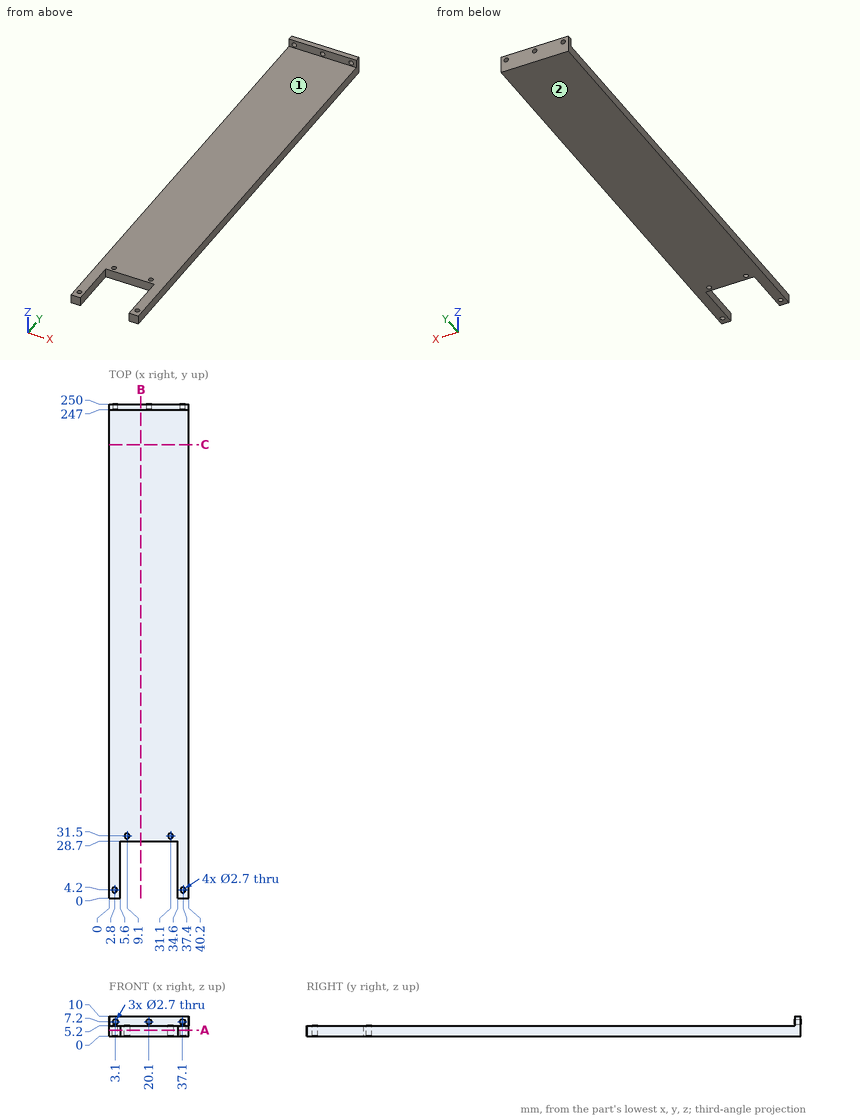
Source: three-view drawing plus pictorial views. Frame: mm from the lowest corner of the part. A direction names the side the tool comes from. Coordinates: 2 decimals unless noted, no trailing zeros. Order: outer loops, then holes, each group sorted by start corner. A loop starts at its lowest first (then second) coordinate and runs counter-clockwise, first axis right, second up.
1) Section B-B (x = 16). Return loops of the section in (y, z), then the cut area to 3 significant figures.
Result sheet:
outline: (28.7, 0) - (250, 0) - (250, 10) - (247, 10) - (247, 5.2) - (28.7, 5.2) - close
area: 1,170 mm2
2) Section A-A (z = 3). Return loops of the section in (x, y).
Result sheet:
outline: (0, 0) - (5.6, 0) - (5.6, 28.7) - (34.6, 28.7) - (34.6, 0) - (40.2, 0) - (40.2, 250) - (0, 250) - close; hole circle Ø2.7 at (2.8, 4.2); hole circle Ø2.7 at (9.1, 31.5); hole circle Ø2.7 at (31.1, 31.5); hole circle Ø2.7 at (37.4, 4.2)
3) Section C-C (y = 229.5). Return loops of the section in (x, z), then the cut area to 3 significant figures.
Result sheet:
outline: (0, 0) - (40.2, 0) - (40.2, 5.2) - (0, 5.2) - close
area: 209 mm2
4) Ray query, probe 1 along Z at (x, y) = (37.1, 248.3); probe 2 along Y at (x, z) = (37.4, 1.1); probe 3 along Y at (x, z) = (9.1, 2.4). Return the intervals inside material, ascending.
Result sheet:
probe 1: z = 0 to 5.85, 8.55 to 10
probe 2: y = 0 to 2.85, 5.55 to 250
probe 3: y = 28.7 to 30.15, 32.85 to 250
5) First-contact query: P1, Ø1.6, axis at x = 19, z = 3.5, coming from the -Y side; P2, Ø6, axis at x = 16, y = 135, coming from the +Z side; P3, Ø5.5, axis at x = 25, z = 8, coming from the -Y side. Flat tips, straight axial feed; report the tip coordinate or a pass-through.
Result sheet:
P1: stops at y = 28.7
P2: stops at z = 5.2
P3: stops at y = 247
6) Set-up query: the marked faces 1 and 2. Return all of +Z, -Z, +X, -X, +Y, -Y with unobstructed straight access to the full face (end or side cutting, diameter ignored); none if empty.
Result sheet:
face 1: +Z, +X, -X, -Y
face 2: -Z, +X, -X, +Y, -Y
